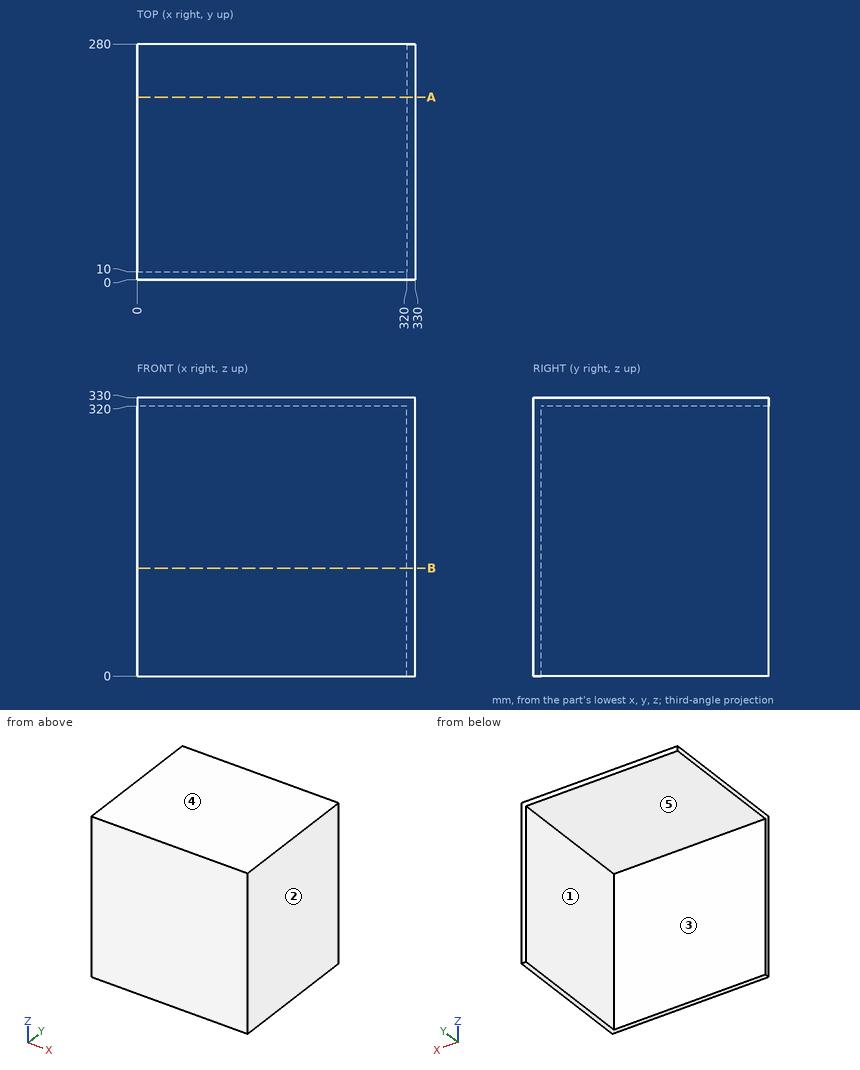
Geometry: see drawing. Coordinates: mm, zero at the bounding-box minimum. A direction names the side the tool comes from. Round coordinates to 2 decimals unless told otherwise and drop trailing zeros. Order: outer loops, then holes, each group sorted by start corner. A loop starts at its lowest first (then second) coordinate and runs counter-clockwise, first axis right, second up. Notation, with made-up numbers: (1, -3) -> (45, -3) arc R24 cw to (45, 10) -> close; hole circle Ø6 at (14.5, -38). An arc over 180 degrees is marked (long way). Answer as CSV lines item,"result".
Item 1: Section A-A, the plane y = 217. Return loops of the section in (x, z), plus the area to 3 significant figures.
A:
outline,"(0, 320) -> (320, 320) -> (320, 0) -> (330, 0) -> (330, 330) -> (0, 330) -> close"
area,"6,500 mm²"
Item 2: Section B-B, the plane z = 128. Return loops of the section in (x, y).
A:
outline,"(0, 0) -> (330, 0) -> (330, 280) -> (320, 280) -> (320, 10) -> (0, 10) -> close"
Item 3: Line query: L1, parallel to Y at x = 306, z = 194.5; L2, parallel to Z at x = 193.5, y = 186.5. Output: solid intervals per line, ascending.
A:
L1,"0 to 10"
L2,"320 to 330"
Item 4: Pin query (flat end, axial travel): pin 1 Ø12 at (x, z) = (286, 45.5) entering from +Y; pin 2 Ø5 at (y, z) = (113.5, 215.5) entering from -X; pin 3 Ø4 at (x, y) = (91, 216) entering from -Z. Return the tip coordinate at first contact, or that it passes through.
A:
pin 1,"y = 10"
pin 2,"x = 320"
pin 3,"z = 320"
Item 5: Pull-direction query (Z, two-part tool) for the marked faces 3, 4 and 5; classes: pulls with the +Z half, pulls with the -Z half, needs draft (parallel to the pull), parting line crosses it, or undercut.
A:
face 3,"needs draft"
face 4,"pulls with the +Z half"
face 5,"pulls with the -Z half"
Item 6: Reachability of the marked faces 1 and 2 from +Z, -Z, +X, -X, +Y, -Y: full face, straight path, thin tool, end or side. Return the list, or none.
A:
face 1,"-Z, -X, +Y"
face 2,"+Z, -Z, +X, +Y, -Y"
